from build123d import *

# Parameters (mm, degrees)
BOSS_EXTRUDE1_DEPTH       = 101.603999992
CUT_EXTRUDE1_DEPTH        = 246.126
SKETCH14_W                = 76.2
SKETCH14_H                = 76.2
SKETCH14_W_2              = 63.5
SKETCH14_H_2              = 63.5
BOSS_EXTRUDE3_DEPTH       = 101.603999992
FILLET1_R                 = 4
M3X0_5_TAPPED_HOLE2_D     = 2.5
M3X0_5_TAPPED_HOLE2_DEPTH = 7.5
M3X0_5_TAPPED_HOLE2_TIP   = 0.751075774
M3X0_5_TAPPED_HOLE1_D     = 2.5
M3X0_5_TAPPED_HOLE1_DEPTH = 7.5
M3X0_5_TAPPED_HOLE1_TIP   = 0.751075774
FILLET2_R                 = 1


with BuildPart() as part:
    # Sketch1 → Boss-Extrude1 (new body)
    with BuildSketch(Plane(origin=(0, 0, 0), x_dir=(1, 0, 0), z_dir=(0, 1, 0))):
        with BuildLine():
            Line((-35.56, -38.1), (35.56, -38.1))
            ThreePointArc((35.56, -38.1), (37.356051224, -37.356051224), (38.1, -35.56))
            Line((38.1, -35.56), (38.1, 35.56))
            ThreePointArc((38.1, 35.56), (37.356051224, 37.356051224), (35.56, 38.1))
            Line((35.56, 38.1), (-35.56, 38.1))
            ThreePointArc((-35.56, 38.1), (-37.356051224, 37.356051224), (-38.1, 35.56))
            Line((-38.1, 35.56), (-38.1, -35.56))
            ThreePointArc((-38.1, -35.56), (-37.356051224, -37.356051224), (-35.56, -38.1))
        make_face()
    extrude(amount=BOSS_EXTRUDE1_DEPTH)

    # Sketch9 → Cut-Extrude1 (cut)
    with BuildSketch(Plane(origin=(0, 101.603999992, 0), x_dir=(1, 0, 0), z_dir=(0, 1, 0))):
        with BuildLine():
            Line((-30.56, -33.1), (30.56, -33.1))
            ThreePointArc((30.56, -33.1), (32.356051224, -32.356051224), (33.1, -30.56))
            Line((33.1, -30.56), (33.1, 30.56))
            ThreePointArc((33.1, 30.56), (32.356051224, 32.356051224), (30.56, 33.1))
            Line((30.56, 33.1), (-30.56, 33.1))
            ThreePointArc((-30.56, 33.1), (-32.356051224, 32.356051224), (-33.1, 30.56))
            Line((-33.1, 30.56), (-33.1, -30.56))
            ThreePointArc((-33.1, -30.56), (-32.356051224, -32.356051224), (-30.56, -33.1))
        make_face()
    extrude(amount=-CUT_EXTRUDE1_DEPTH, mode=Mode.SUBTRACT)

    # Sketch14 → Boss-Extrude3 (add)
    with BuildSketch(Plane(origin=(0, 101.603999992, 0), x_dir=(1, 0, 0), z_dir=(0, 1, 0))):
        Rectangle(SKETCH14_W, SKETCH14_H)
        Rectangle(SKETCH14_W_2, SKETCH14_H_2, mode=Mode.SUBTRACT)
    extrude(amount=-BOSS_EXTRUDE3_DEPTH)

    # Fillet1
    fillet1_edges = [part.edges().sort_by_distance(p)[0] for p in [
        (38.1, 50.801999996, -38.1),
        (38.1, 50.801999996, 38.1),
        (-38.1, 50.801999996, 38.1),
        (-38.1, 50.801999996, -38.1),
    ]]
    fillet(fillet1_edges, radius=FILLET1_R)

    # M3x0.5 Tapped Hole2
    with Locations(Plane(origin=(0, 101.603999992, 0), x_dir=(1, 0, 0), z_dir=(0, 1, 0))):
        with Locations((-34.1, 34.1), (34.1, 34.1), (34.1, -34.100008), (-34.1, -34.100008), (-34.95, 0), (34.94999995, 0), (0, -34.95), (0, 34.95)):
            Hole(M3X0_5_TAPPED_HOLE2_D / 2, depth=M3X0_5_TAPPED_HOLE2_DEPTH)
            with Locations((0, 0, -(M3X0_5_TAPPED_HOLE2_DEPTH + M3X0_5_TAPPED_HOLE2_TIP / 2))):  # 118° drill point
                Cone(0, M3X0_5_TAPPED_HOLE2_D / 2, M3X0_5_TAPPED_HOLE2_TIP, mode=Mode.SUBTRACT)

    # M3x0.5 Tapped Hole1
    with Locations(Plane(origin=(0, 0, 0), x_dir=(-1, 0, 0), z_dir=(0, -1, 0))):
        with Locations((-34.100008, 34.1), (34.1, 34.1), (34.1, -34.1), (-34.100008, -34.1), (-34.95, 0), (0, 34.95), (34.95, 0), (0, -34.94999995)):
            Hole(M3X0_5_TAPPED_HOLE1_D / 2, depth=M3X0_5_TAPPED_HOLE1_DEPTH)
            with Locations((0, 0, -(M3X0_5_TAPPED_HOLE1_DEPTH + M3X0_5_TAPPED_HOLE1_TIP / 2))):  # 118° drill point
                Cone(0, M3X0_5_TAPPED_HOLE1_D / 2, M3X0_5_TAPPED_HOLE1_TIP, mode=Mode.SUBTRACT)

    # Fillet2
    fillet2_edges = [part.edges().sort_by_distance(p)[0] for p in [
        (31.75, 50.801999996, 31.75),
        (-31.75, 50.801999996, 31.75),
        (-31.75, 50.801999996, -31.75),
        (31.75, 50.801999996, -31.75),
    ]]
    fillet(fillet2_edges, radius=FILLET2_R)


solid = part.part
Work out the finished part from the listing and answer in its coordinate system (mm). A direction names the side the tool comes from. Give positions to 0.01 mm unless a question says otherwise; leave off trailing zeros. Loops run counter-clockwise (first coordinate to the right, second up) from the corner with the lowest first, then second, coordinate; pieces in that order, holes last. Notation, with made-up numbers: M 41.5,76 L 85.5,76 A15 ccw 85.5,96 Z; hole C 69,-7.5 d11. An arc over 180 degrees is marked long. Use CSV: the item, a comma, the result in double quotes.
1) Consider L1, parallel to Z at x = -26.5, y = 54.5; L2, parallel to X at y = 5.75, z = 34.95. Determine where each line is inside the solid, lowest interval first.
Answer:
L1,"-38.1 to -31.75, 31.75 to 38.1"
L2,"-38.01 to -35.02, -33.18 to -1.25, 1.25 to 33.18, 35.02 to 38.01"
2) Find section A-A on x = 7. Write down the section's boundary in (y, z), plus the area to 3 significant figures.
Answer:
outline,"M 0,-38.1 L 101.6,-38.1 L 101.6,-31.75 L 0,-31.75 Z; M 0,31.75 L 101.6,31.75 L 101.6,38.1 L 0,38.1 Z"
area,"1,290 mm^2"
3) Given P1, Ø3, axis at x = -34.1, z = 34.1, coming from the -Y side; P2, Ø1.5, axis at x = -34.1, z = -34.1, coming from the +Y side; P3, Ø1.5, axis at x = -34.1, z = -34.1, coming from the -Y side; P4, Ø2, axis at x = -34.1, z = 34.1, coming from the +Y side, each flat-ended and moving along its own axis, determine where each tip first touches the part or whether it passes through.
Answer:
P1,"y = 0"
P2,"y = 93.8"
P3,"y = 7.8"
P4,"y = 93.95"
4) Find section B-B on y = 28. Write down the section's boundary in (x, z), plus the area to 3 significant figures.
Answer:
outline,"M -38.1,-34.1 A4 ccw -34.1,-38.1 L 34.1,-38.1 A4 ccw 38.1,-34.1 L 38.1,34.1 A4 ccw 34.1,38.1 L -34.1,38.1 A4 ccw -38.1,34.1 Z; hole M -31.75,-30.75 A1 ccw -30.75,-31.75 L 30.75,-31.75 A1 ccw 31.75,-30.75 L 31.75,30.75 A1 ccw 30.75,31.75 L -30.75,31.75 A1 ccw -31.75,30.75 Z"
area,"1,760 mm^2"
5) Which of the six approach directions +Z, -Z, +X, -X, +Y, -Y give full straight-line access (tool end or side, diameter ignored) to faces 1 (the flat face through (38.1, 50, 0)), 2 (the cylindrical face through (-0.27, 3.8, -33.73)), 3 (the cylindrical face through (-33.7, 97.8, -0.05)), 4 (the cylindrical face through (36.897, 50.091, -36.959)), 5 (the flat face through (0, 52, -31.75))?
Answer:
face 1,"+Z, -Z, +X, +Y, -Y"
face 2,"-Y"
face 3,"+Y"
face 4,"-Z, +X, +Y, -Y"
face 5,"+Y, -Y"
6) Determine the mould class of faces 6 (the flat face through (0, 50, -38.1)), 7 (the cylindrical face through (33.11, 3.8, -33.34)), 8 (the cylindrical face through (-36.959, 50.091, -36.897)) for opening direction X: released by +X, released by -X, zero draft, split by the parting line, or undercut.
Answer:
face 6,"zero draft"
face 7,"undercut"
face 8,"released by -X"
7) Find section C-C on z = 29.5. Write down the section's boundary in (x, y).
Answer:
outline,"M -38.1,0 L -31.75,0 L -31.75,101.6 L -38.1,101.6 Z; M 31.75,0 L 38.1,0 L 38.1,101.6 L 31.75,101.6 Z"
